For this review, take the finished solid that the model builds, in its own axes (mm). Face numbers are marked on the shaded views. A direction names the side the tool comes from. Round coordinates to 2 decimals unless told otherwise and drop trailing zeros. Order: outer loops, then holes, each group sorted by start corner. A loop starts at its lowest first (then second) coordinate and runs counter-clockwise, first axis right, second up. Notation, with made-up numbers: (-18.75, 56) - (-2.75, 56) arc R16 ccw to (-2.75, 83) - close; hole circle Ø7 at (-11.75, 57). An arc over 180 degrees is marked (long way). One line per item, written item: value.
```python
from build123d import *

# Parameters (mm, degrees)
SKETCH1_R           = 1.5
BOSS_EXTRUDE1_DEPTH = 3
SKETCH2_W           = 3
SKETCH2_H           = 3
CUT_EXTRUDE1_DEPTH  = 3
FILLET1_R           = 3


with BuildPart() as part:
    # Sketch1 → Boss-Extrude1 (new body)
    with BuildSketch(Plane(origin=(0, 0, 0), x_dir=(0, 0, -1), z_dir=(1, 0, 0))):
        Polygon((-12.5, -7.5), (-12.5, -3), (-9.5, -3), (-9.5, 3), (-12.5, 3), (-12.5, 7.5), (12.5, 7.5), (12.5, -7.5), align=None)
        Circle(SKETCH1_R, mode=Mode.SUBTRACT)
    extrude(amount=BOSS_EXTRUDE1_DEPTH)

    # Sketch2 → Cut-Extrude1 (cut)
    with BuildSketch(Plane(origin=(3, 0, 0), x_dir=(0, 0, -1), z_dir=(1, 0, 0))):
        with Locations((-5, 5)):
            Rectangle(SKETCH2_W, SKETCH2_H)
        with Locations((-5, -5)):
            Rectangle(SKETCH2_W, SKETCH2_H)
    extrude(amount=-CUT_EXTRUDE1_DEPTH, mode=Mode.SUBTRACT)

    # Fillet1
    fillet1_edges = [part.edges().sort_by_distance(p)[0] for p in [
        (1.5, -7.5, -12.5),
        (1.5, 7.5, -12.5),
    ]]
    fillet(fillet1_edges, radius=FILLET1_R)


solid = part.part
```
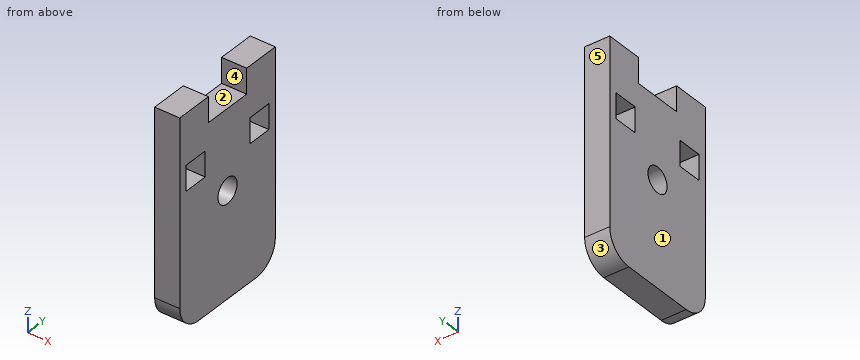
Item 1: Machinability: for the marked faces 4 and 5, which of the approach directions +Z, -Z, +X, -X, +Y, -Y give a long, thin tool a straight path to every point of the face, cutting with its end or side? Answer none if there is none.
Returned:
face 4: +Z, +X, -X
face 5: +Z, -Z, +X, -X, +Y
Item 2: Take a section at C-C (x = 1.1). Write out the cut boundary in (y, z).
Returned:
outline: (-7.5, -9.5) arc R3 ccw to (-4.5, -12.5) - (4.5, -12.5) arc R3 ccw to (7.5, -9.5) - (7.5, 12.5) - (3, 12.5) - (3, 9.5) - (-3, 9.5) - (-3, 12.5) - (-7.5, 12.5) - close; hole (-6.5, 3.5) - (-3.5, 3.5) - (-3.5, 6.5) - (-6.5, 6.5) - close; hole circle Ø3 at (0, 0); hole (3.5, 3.5) - (6.5, 3.5) - (6.5, 6.5) - (3.5, 6.5) - close
Item 3: Take a section at A-A (z = 0). Write out the cut boundary in (x, y).
Returned:
outline: (0, -7.5) - (3, -7.5) - (3, -1.5) - (0, -1.5) - close; (0, 1.5) - (3, 1.5) - (3, 7.5) - (0, 7.5) - close
Item 4: Take a section at B-B (y = 0). Write out the cut boundary in (x, z), plus the area to 3 significant figures.
Returned:
outline: (0, -12.5) - (3, -12.5) - (3, -1.5) - (0, -1.5) - close; (0, 1.5) - (3, 1.5) - (3, 9.5) - (0, 9.5) - close
area: 57.0 mm^2
Item 5: The part is to be moulded in two halves that separate along Y. For the marked faces 1, 2 and 3, say which applies: +Y half, -Y half, draft (parallel to the pull), parting line (faces both ways), or undercut.
Returned:
face 1: draft
face 2: undercut
face 3: +Y half
Item 6: Wall thickness on line 1 (Y direction, x = 2.1, z = 5.5); line 2 (Y direction, x = 1.8, z = 0); line 3 (Z direction, x = 1.1, y = 4.5): over which ranges is each line inside the solid? List them lowest first.
Returned:
line 1: -7.5 to -6.5, -3.5 to 3.5, 6.5 to 7.5
line 2: -7.5 to -1.5, 1.5 to 7.5
line 3: -12.5 to 3.5, 6.5 to 12.5
Item 7: Take a section at D-D (y = -2.25). Write out the cut boundary in (x, z).
Returned:
outline: (0, -12.5) - (3, -12.5) - (3, 9.5) - (0, 9.5) - close
